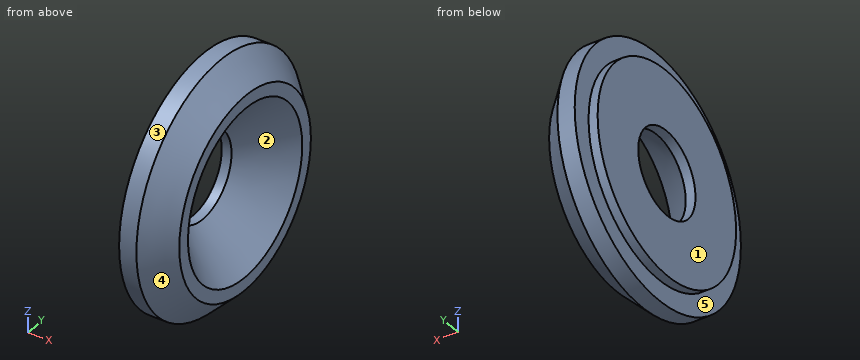
```python
from build123d import *

# Parameters (mm, degrees)
HOLE1_D           = 10.5
HOLE1_DEPTH       = 16.51
HOLE1_CSINK_D     = 20.955
HOLE1_CSINK_ANGLE = 90
HOLE1_TIP         = 3.15451825


with BuildPart() as part:
    # Sketch1 → Revolve1 (revolve)
    with BuildSketch(Plane.XY):
        Polygon((461.35385273, 245.11), (461.35385273, 232.41), (467.794592233, 232.41), (467.794592233, 244.475), (464.619592233, 247.65), (462.47885273, 247.65), (462.47885273, 245.11), align=None)
    revolve(axis=Axis((443.287790535, 232.41, 0), (1, 0, 0)))

    # Hole1
    with Locations(Plane(origin=(467.794592233, 0, 0), x_dir=(0, 0, -1), z_dir=(1, 0, 0))):
        with Locations((0, 232.41)):
            CounterSinkHole(HOLE1_D / 2, HOLE1_CSINK_D / 2, depth=HOLE1_DEPTH, counter_sink_angle=HOLE1_CSINK_ANGLE)
            with Locations((0, 0, -(HOLE1_DEPTH + HOLE1_TIP / 2))):  # 118° drill point
                Cone(0, HOLE1_D / 2, HOLE1_TIP, mode=Mode.SUBTRACT)


solid = part.part
```
Design review of the part built by this model. Coordinates are the model's own, in mm. Face numbers are marked on the shaded views. A direction names the side the tool comes from. Coordinates: 2 decimals unless noted, no trailing zeros. Loops run counter-clockwise (first coordinate to the right, second up) from the corner with the lowest first, then second, coordinate; pieces in that order, holes last. Notation, with made-up numbers: (-18, -14) - (30, -14) arc R30 cw to (30, 16) - close; hole circle Ø8 at (2, 63). An arc over 180 degrees is marked (long way). Use CSV: the item, a comma, the result in double quotes. Start each with the question number.
1) The part is to be moulded in two halves that separate along Y. For the marked faces 1, 2 and 3, say which applies: +Y half, -Y half, draft (parallel to the pull), parting line (faces both ways), or undercut.
2) For pin 1 Ø1 at (x, y) = (465, 225.5) entering from -Z; pin 2 Ø1 at (x, z) = (464.5, -12) entering from +Y; pin 3 Ø3 at (x, y) = (465, 229) entering from -Z; pin 4 Ø6.5 at (y, z) = (232.41, 0) entering from +X, all flat-tipped, find the tip position at first contact; note any pin that passes through.
3) Wall thickness on L1, parallel to Z at x = 462.2, y = 232.41; L2, parallel to Y at x = 466.75, z = 8.5; L3, parallel to Y at x = 464.5, z = -0.5: over which ranges is each line inside the solid? List them lowest first. Write a range as from..to.
4) Consider section C-C on x = 462. Write out the cut boundary in (y, z).
5) Tool access review of the marked faces 4 and 5: name each direction out of +Z, -Z, +X, -X, +Y, -Y from which nothing blocks a thin tool from reaching the whole face with its end or side.
6) Consider section D-D on x = 466.75. Write out the cut boundary in (y, z).
Geometry says:
1,face 1,"draft"
1,face 2,"undercut"
1,face 3,"parting line"
2,pin 1,"z = -13.74"
2,pin 2,"y = 242.41"
2,pin 3,"z = -15.11"
2,pin 4,"through"
3,L1,"-12.7..-5.25, 5.25..12.7"
3,L2,"222.43..228.32, 236.5..242.39"
3,L3,"217.18..225.24, 239.58..247.64"
4,outline,"circle Ø25.4 at (232.41, 0); hole circle Ø10.5 at (232.41, 0)"
5,face 4,"+X"
5,face 5,"-X"
6,outline,"circle Ø26.22 at (232.41, 0); hole circle Ø18.87 at (232.41, 0)"
